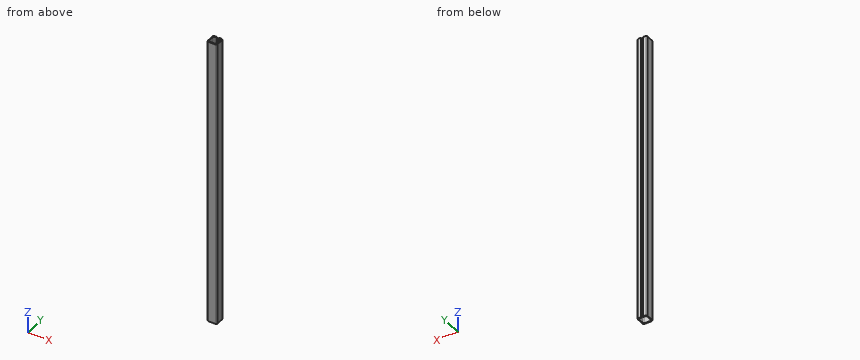
```python
from build123d import *

# Parameters (mm, degrees)
DODANIE_WYCI_GNI_CIE1_DEPTH = 600


with BuildPart() as part:
    # Szkic1 → Dodanie-wyciągnięcie1 (new body)
    with BuildSketch(Plane.XY):
        with BuildLine():
            Line((-10, -7), (-10, 7))
            ThreePointArc((-10, 7), (-9.121320344, 9.121320344), (-7, 10))
            Line((-7, 10), (-2, 10))
            Line((-2, 10), (-2, 8))
            Line((-2, 8), (-6, 8))
            ThreePointArc((-6, 8), (-7.414213562, 7.414213562), (-8, 6))
            Line((-8, 6), (-8, -6))
            ThreePointArc((-8, -6), (-7.414213562, -7.414213562), (-6, -8))
            Line((-6, -8), (6, -8))
            ThreePointArc((6, -8), (7.414213562, -7.414213562), (8, -6))
            Line((8, -6), (8, 6))
            ThreePointArc((8, 6), (7.414213562, 7.414213562), (6, 8))
            Line((6, 8), (2, 8))
            Line((2, 8), (2, 10))
            Line((2, 10), (7, 10))
            ThreePointArc((7, 10), (9.121320344, 9.121320344), (10, 7))
            Line((10, 7), (10, -7))
            ThreePointArc((10, -7), (9.121320344, -9.121320344), (7, -10))
            Line((7, -10), (-7, -10))
            ThreePointArc((-7, -10), (-9.121320344, -9.121320344), (-10, -7))
        make_face()
    extrude(amount=DODANIE_WYCI_GNI_CIE1_DEPTH)


solid = part.part
```
Verification items for the finished model (mm, model axes). Coordinates: 2 decimals unless noted, no trailing zeros. Write each loop counter-clockwise with the first axis right and the second up, starting at its lowest first coordinate (ties: lowest second). Pieces come first, ordered by that corner, then holes. Notation, with made-up numbers: (-15.75, 29) - (0.25, 29) arc R26 ccw to (0.25, 59) - close; hole circle Ø7 at (16.5, 77.5). An arc over 180 degrees is marked (long way). One line per question, with ' | ' between items. Start each with the question number.
1. Section check A-A (y = 0.5). Enter the section's corners in (x, z), plus the area to 3 significant figures.
2. Section check B-B (z = 308.5). Enter the section's corners in (x, y).
3. Material ranges on line 1 along X through (y, z) = (-0.25, 244); line 2 along Y through (x, z) = (-7.75, 280), recorded low to high.
4. Gauge pin test, flat ends, axial feed: P1, Ø1, axis at y = 8.5, z = 291.5, coming from the +X side; P2, Ø0.6, axis at y = 8.5, z = 363, coming from the -X side. Record the tip position at first contact, or that the pin passes through.
Computed values:
1) outline: (-10, 0) - (-8, 0) - (-8, 600) - (-10, 600) - close; (8, 0) - (10, 0) - (10, 600) - (8, 600) - close | area: 2,400 mm²
2) outline: (-10, -7) arc R3 ccw to (-7, -10) - (7, -10) arc R3 ccw to (10, -7) - (10, 7) arc R3 ccw to (7, 10) - (2, 10) - (2, 8) - (6, 8) arc R2 cw to (8, 6) - (8, -6) arc R2 cw to (6, -8) - (-6, -8) arc R2 cw to (-8, -6) - (-8, 6) arc R2 cw to (-6, 8) - (-2, 8) - (-2, 10) - (-7, 10) arc R3 ccw to (-10, 7) - close
3) line 1: -10 to -8, 8 to 10 | line 2: -9.9 to -6.97, 6.97 to 9.9
4) P1: x = 9.83 | P2: x = -9.75
